Drawing for the job (mm, zero at the part's lowest x, y, z). Give positions to 0.01 mm unless a question says otherwise; leave off trailing zeros. Loops run counter-clockwise (first coordinate to the right, second up) from the corner with the lowest first, then second, coordinate; pieces in that order, holes last. Notation, with made-up numbers: (-21.75, 33.5) -> (-9.75, 33.5) arc R13 cw to (-9.75, 48.5) -> close; hole circle Ø3 at (-12.75, -22). An arc over 180 degrees is marked (long way). Write item = value, one per line.
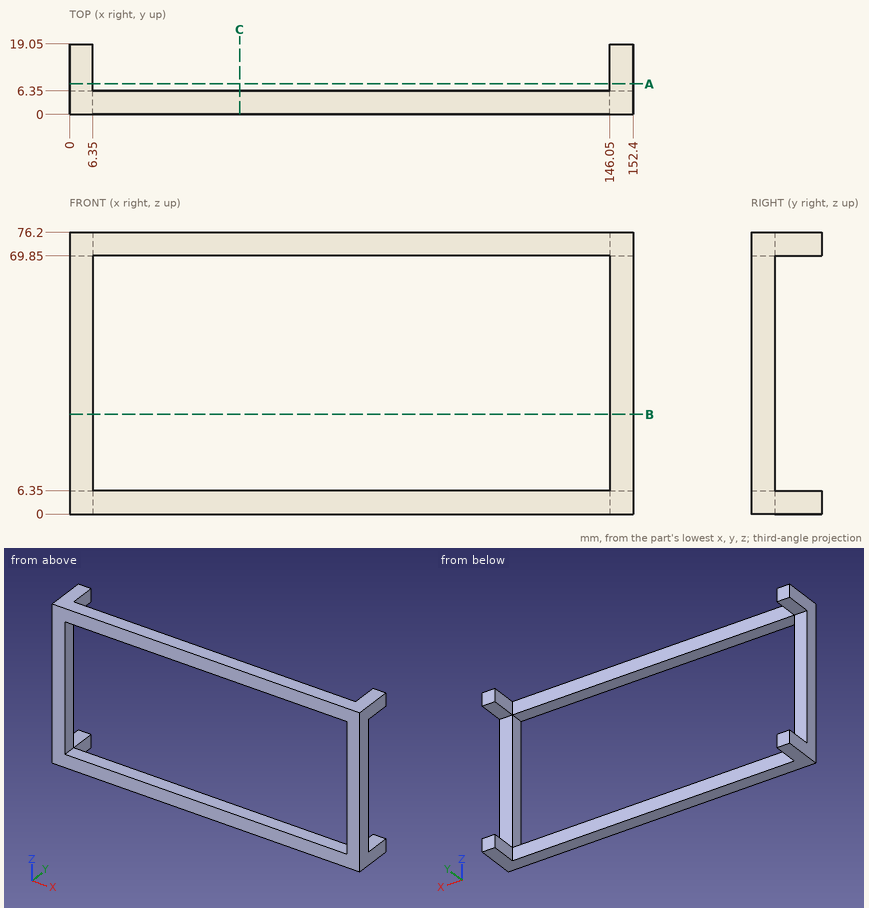
1) Slice it at B-B, the plane z = 27. List the corners of the cut face in (x, y), and give its area (3 significant figures).
Resolved:
outline = (0, 0) -> (6.35, 0) -> (6.35, 6.35) -> (0, 6.35) -> close; (146.05, 0) -> (152.4, 0) -> (152.4, 6.35) -> (146.05, 6.35) -> close
area = 80.6 mm²
2) Drill centre lines: line 1 along X through (y, z) = (3.5, 65); line 2 along Z through (x, y) = (52, 3.75). Where is each one in solid material? Low to high. Write a range as [from, to].
Resolved:
line_1 = [0, 6.35], [146.05, 152.4]
line_2 = [0, 6.35], [69.85, 76.2]
3) Slice it at A-A, the plane y = 8.25. List the corners of the cut face in (x, z).
Resolved:
outline = (0, 0) -> (6.35, 0) -> (6.35, 6.35) -> (0, 6.35) -> close; (0, 69.85) -> (6.35, 69.85) -> (6.35, 76.2) -> (0, 76.2) -> close; (146.05, 0) -> (152.4, 0) -> (152.4, 6.35) -> (146.05, 6.35) -> close; (146.05, 69.85) -> (152.4, 69.85) -> (152.4, 76.2) -> (146.05, 76.2) -> close
4) Slice it at C-C, the plane x = 46. List the corners of the cut face in (y, z).
Resolved:
outline = (0, 0) -> (6.35, 0) -> (6.35, 6.35) -> (0, 6.35) -> close; (0, 69.85) -> (6.35, 69.85) -> (6.35, 76.2) -> (0, 76.2) -> close
5) Drop flat-ended pins along their axis: P1, Ø3, axis at x = 150, z = 29, coming from the +Y side; P2, Ø10, axis at x = 125, z = 12.5, coming from the -Y side (1 decimal). Give the stop position or say it passes through.
Resolved:
P1 = 6.35
P2 = through
